Could you check a few things on this model? Use its own coordinates, in mm. Face numbers are marked on the shaded views. Round coordinates to 2 decimals unless told otherwise and drop trailing zeros. Loops run counter-clockwise (first coordinate to the right, second up) from the corner with the lowest first, then second, coordinate; pieces in that order, holes last. Notation, with made-up numbers: (-3, 79.5) - (20, 79.5) arc R30 ccw to (20, 115.5) - close; hole circle Ø10 at (-26, 23). An arc over 180 degrees is marked (long way). Put each result on its own line as item: value. Start each with the question number.
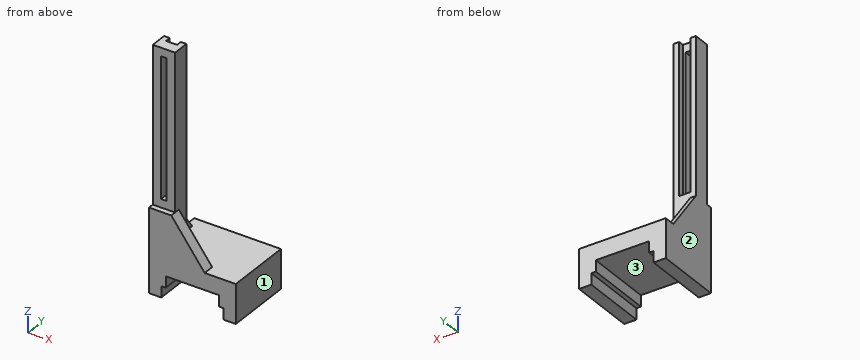
from build123d import *

# Parameters (mm, degrees)
F1_DEPTH  = 38.1
F2_W      = 71.12
F2_H      = 27.39084
F3_DEPTH  = 50.8
F4_W      = 25.4
F4_H      = 19.05
F5_DEPTH  = 228.6
F6_W      = 25.4
F6_H      = 50.8
F7_DEPTH  = 12.7
F9_DEPTH  = 6.35
F10_W     = 12.7
F10_H     = 165.1
F11_DEPTH = 6.35
F12_W     = 6.35
F12_H     = 158.75
F13_DEPTH = 25.4
F14_W     = 12.7
F14_H     = 25.4
F14_H_2   = 6.35
F15_DEPTH = 6.35


with BuildPart() as f1:
    # F0 (on Front) → F1 (new body, symmetric)
    with BuildSketch(Plane.XZ):
        Polygon((30.48, -22.225), (49.53, -22.225), (49.53, 22.225), (-49.53, 22.225), (-49.53, -22.225), (-30.48, -22.225), (-30.48, 3.175), (30.48, 3.175), align=None)
    extrude(amount=F1_DEPTH, both=True)

    # F2 (on Front) → F3 (cut, symmetric)
    with BuildSketch(Plane.XZ):
        with Locations((0, -23.22042)):
            Rectangle(F2_W, F2_H)
    extrude(amount=F3_DEPTH, both=True, mode=Mode.SUBTRACT)

    # F4 (on face) → F5 (join)
    with BuildSketch(Plane.XY.offset(22.225)):
        with Locations((-36.83, -22.225)):
            Rectangle(F4_W, F4_H)
    extrude(amount=F5_DEPTH)

    # F6 (on face) → F7 (join)
    with BuildSketch(Plane.XZ.offset(38.1)):
        with Locations((-36.83, 47.625)):
            Rectangle(F6_W, F6_H)
        Polygon((-24.13, 73.025), (-24.13, 22.225), (13.97, 22.225), align=None)
    extrude(amount=-F7_DEPTH)

    # F8 (on face) → F9 (join)
    with BuildSketch(Plane(origin=(-49.53, 0, 0), x_dir=(0, -1, 0), z_dir=(-1, 0, 0))):
        Polygon((-25.4, 22.225), (12.7, 22.225), (12.7, 73.025), align=None)
    extrude(amount=-F9_DEPTH)

    # F10 (on face) → F11 (cut)
    with BuildSketch(Plane(origin=(0, -12.7, 0), x_dir=(-1, 0, 0), z_dir=(0, 1, 0))):
        with Locations((36.83, 161.925)):
            Rectangle(F10_W, F10_H)
    extrude(amount=-F11_DEPTH, mode=Mode.SUBTRACT)

    # F12 (on face) → F13 (cut)
    with BuildSketch(Plane(origin=(0, -19.05, 0), x_dir=(-1, 0, 0), z_dir=(0, 1, 0))):
        with Locations((36.83, 161.925)):
            Rectangle(F12_W, F12_H)
    extrude(amount=-F13_DEPTH, mode=Mode.SUBTRACT)

    # F14 (on face) → F15 (cut)
    with BuildSketch(Plane(origin=(0, -12.7, 0), x_dir=(-1, 0, 0), z_dir=(0, 1, 0))):
        with Locations((36.83, 250.825)):
            Rectangle(F14_W, F14_H)
        with Locations((36.83, 241.3)):
            Rectangle(F14_W, F14_H_2)
    extrude(amount=-F15_DEPTH, mode=Mode.SUBTRACT)


solid = f1.part
Item 1: Thinking about a two-plate mould opening in X: for the marked faces 1, 2 and 3, which applies, released by +X, released by -X, zero draft, split by the parting line, or undercut?
Item 2: Suppose I cut it at C-C, the plane x = -27. List the corners of the cut face in (y, z) for me (3 decimals), then the cut area to 3 significant figures.
Item 3: Will these pins go through, and if not, where does the flat tip stop? P1, Ø7, axis at y = -15.5, z = 167.5, coming from the +X side; P2, Ø8, axis at x = 39, y = 9.5, coming from the +Z side (3 decimals); P3, Ø10, axis at x = -30.5, y = 16.5, coming from the -Z side (3 decimals); P4, Ø10, axis at y = -5, z = 183, coming from the -X side.
Item 4: I need wall thicknesses on line 1 (X direction, y = 14, z = -4.5); line 2 (X direction, y = -30, z = 88) (3 decimals); line 3 (Z direction, x = -13, y = 25) (3 decimals). Which ranges of each line are inside material? Lowest first, please. Write a range as from..to.
Item 5: Suppose I cut it at A-A, the plane z = 0. List the corners of the cut face in (x, y) for me, then the cut area to 3 significant figures.
Item 6: Suppose I cut it at D-D, the plane z = 94. List the corners of the cut face in (x, y) for me (3 decimals).
Item 7: Suppose I cut it at B-B, the plane y = 32.5. List the corners of the cut face in (x, z) for me (3 decimals).
Numbers:
1. face 1: released by +X
1. face 2: released by -X
1. face 3: undercut
2. outline: (-38.1, 3.175) - (38.1, 3.175) - (38.1, 22.225) - (-12.7, 22.225) - (-12.7, 250.825) - (-31.75, 250.825) - (-31.75, 73.025) - (-38.1, 73.025) - close
2. area: 6,130 mm^2
3. P1: x = -24.13
3. P2: z = 22.225
3. P3: z = -9.525
3. P4: through
4. line 1: -49.53..-30.48, 30.48..49.53
4. line 2: -49.53..-40.005, -33.655..-24.13
4. line 3: 3.175..22.225
5. outline: (-49.53, -38.1) - (-30.48, -38.1) - (-30.48, 38.1) - (-49.53, 38.1) - close; (30.48, -38.1) - (49.53, -38.1) - (49.53, 38.1) - (30.48, 38.1) - close
5. area: 2,900 mm^2
6. outline: (-49.53, -31.75) - (-40.005, -31.75) - (-40.005, -19.05) - (-43.18, -19.05) - (-43.18, -12.7) - (-49.53, -12.7) - close; (-33.655, -31.75) - (-24.13, -31.75) - (-24.13, -12.7) - (-30.48, -12.7) - (-30.48, -19.05) - (-33.655, -19.05) - close
7. outline: (-49.53, -22.225) - (-35.56, -22.225) - (-35.56, -9.525) - (-30.48, -9.525) - (-30.48, 3.175) - (30.48, 3.175) - (30.48, -9.525) - (35.56, -9.525) - (35.56, -22.225) - (49.53, -22.225) - (49.53, 22.225) - (-49.53, 22.225) - close
